```python
from build123d import *

# Parameters (mm, degrees)
SKETCH_1_R      = 12.5
SKETCH_1_R_2    = 9.4
EXTRUDE_1_DEPTH = 6
SKETCH_2_R      = 12.5
SKETCH_2_R_2    = 5
EXTRUDE_2_DEPTH = 1
CHAMFER_1_SIZE  = 1


with BuildPart() as part:
    # 草图1 → 凸台-拉伸1 (new body)
    with BuildSketch(Plane.XY):
        Circle(SKETCH_1_R)
        Circle(SKETCH_1_R_2, mode=Mode.SUBTRACT)
    extrude(amount=EXTRUDE_1_DEPTH)

    # 草图2 → 凸台-拉伸2 (add)
    with BuildSketch(Plane.XY.offset(6)):
        Circle(SKETCH_2_R)
        Circle(SKETCH_2_R_2, mode=Mode.SUBTRACT)
    extrude(amount=EXTRUDE_2_DEPTH)

    # 倒角1
    chamfer_1_edges = [part.edges().sort_by_distance(p)[0] for p in [
        (-12.5, 0, 7),
    ]]
    chamfer(chamfer_1_edges, length=CHAMFER_1_SIZE)


solid = part.part
```
Part model, mm, in its own coordinate system. A direction names the side the tool comes from. Round coordinates to 2 decimals unless told otherwise and drop trailing zeros. Order: outer loops, then holes, each group sorted by start corner. A loop starts at its lowest first (then second) coordinate and runs counter-clockwise, first axis right, second up. Notation, with made-up numbers: M 46.5,88.5 L 96.5,88.5 A22 ccw 96.5,116.5 Z; hole C -6,-8.75 d9. An arc over 180 degrees is marked long. Answer in a Markdown table with one row per item. Add a question column.
Q1. 3-axis set-ups, long thin cutter, end or side, ignore diameter. For faces 5 (the face through (-2.038, -9.176, 2.958)), 6 (the face through (5, -2, 7)): which of +Z, -Z, +X, -X, +Y, -Y reach the whole face in a straight line?
Q2. Cut at C-C on z = 2.75. Give the cut face in (x, y), and give its area (3 significant figures).
Q3. Mould opens along Y. For faces 1 (the face through (-1.08, -4.88, 6.49)), 2 (the face through (-4.7, 8.4, 0)), 3 (the face through (4, -4, 6)), 4 (the face through (11.923, 3.755, 2.958)) say: +Y half, -Y half, draft (parallel to the pull), parting line (faces both ways), or undercut.
Q4. Pin check, flat tips, straight feed: pin 1 (9.5 mm diameter, centred on x = -0.5, y = -1, fed in from -Z); pin 2 (4 mm diameter, centred on y = -6.5, z = 2.5, fed in from +X). Stop position of each tip, or through.
Q5. Wall check: L1, parallel to Y at x = 0, z = 4.3; L2, parallel to Z at x = -3.25, y = 5.75; L3, parallel to Y at x = 7.75, z = 3.5. Give the ranges that are in metal, low to high. Write a range as from..to.
Q6. Cut at A-A on y = 0. Give the cut face in (x, z).
Established:
| question | item | result |
|---|---|---|
| 1 | face 5 | -Z |
| 1 | face 6 | +Z, +X, -X, +Y, -Y |
| 2 | outline | C 0,0 d25; hole C 0,0 d18.8 |
| 2 | area | 213 mm2 |
| 3 | face 1 | undercut |
| 3 | face 2 | draft |
| 3 | face 3 | undercut |
| 3 | face 4 | parting line |
| 4 | pin 1 | stops at z = 6 |
| 4 | pin 2 | stops at x = 11.66 |
| 5 | L1 | y = -12.5..-9.4, 9.4..12.5 |
| 5 | L2 | z = 6..7 |
| 5 | L3 | y = -9.81..-5.32, 5.32..9.81 |
| 6 | outline | M -12.5,0 L -9.4,0 L -9.4,6 L -5,6 L -5,7 L -11.5,7 L -12.5,6 Z; M 5,6 L 9.4,6 L 9.4,0 L 12.5,0 L 12.5,6 L 11.5,7 L 5,7 Z |
